Check sheet for the modelled part. Datum: model origin and axes. Units: mm. A direction names the side the tool comes from. Coordinates: 2 decimals unless noted, no trailing zeros. Loops run counter-clockwise (first coordinate to the right, second up) from the corner with the lowest first, then second, coordinate; pieces in that order, holes last. Notation, with made-up numbers: M 74,-19.75 L 89,-19.75 A17 ccw 89,-9.75 Z; hole C 41.25,51.25 d7. An arc over 180 degrees is marked long. Use CSV: the item, a comma, the result in double quotes. Start each with the question number.
(1) Go/stop test with flat-tipped pins: pin 1 Ø1.4 at (x, y) = (-67.5, -0.25) entering from -Z; pin 2 Ø1.5 at (x, z) = (-87.5, 3.5) entering from -Y; pin 3 Ø2.5 at (y, z) = (-21.5, 3) entering from -X; pin 4 Ø1.5 at (x, z) = (-59.5, 2.5) entering from -Y. Record where each tip stops, or that it passes through.
(2) Section check B-B on x = -64. Record the cut outline in (y, z), and give its area (3 significant figures).
(3) Set-up check for faces 1 (the flat face through (-34, -19.8, 2)), 2 (the flat face through (-1, 0, 5)), 3 (the flat face through (30, -22, 2)), 4 (the flat face through (-30.1, 22, 2)), 5 (the flat face through (82.45, -18, 2)): record each of +Z, -Z, +X, -X, +Y, -Y from which the full face is reachable in a straight line by a thin tool's end or side.
(4) Section check A-A on z = 2.4. Give the number of separate pieces and of enclosed holes in the cut face, and give its area (3 significant figures).
(5) Scan lines: line 1 (Y direction, x = 67.5, z = 3.9); line 2 (Y direction, x = -78, z = 0.7); line 3 (Y direction, x = -1.5, z = 1.85). Record each from-to range of solid material in increasing order.
Autodesk Inventor part; units mm, degrees
ref_plane "YZ Plane" through (0, 0, 0) normal (1, 0, 0) x (0, 1, 0)
ref_plane "XZ Plane" through (0, 0, 0) normal (0, 1, 0) x (-1, 0, 0)
ref_plane "XY Plane" through (0, 0, 0) normal (0, 0, 1) x (1, 0, 0)
sketch "Sketch1" plane through (0, 0, 0) normal (0, 0, 1) x (1, 0, 0)
  line L0 (-89.9, -25) -> (89.9, -25)
  line L1 (89.9, -25) -> (89.9, 25)
  line L2 (89.9, 25) -> (-89.9, 25)
  line L3 (-89.9, 25) -> (-89.9, -25)
  line L4 (-89.9, -25) -> (89.9, 25) construction
  line L5 (89.9, -25) -> (-89.9, 25) construction
  line L6 (46.5, 12.25) -> (67.5, 12.25) construction
  line L7 (67.5, 12.25) -> (67.5, -0.25) construction
  line L8 (67.5, -0.25) -> (46.5, -0.25) construction
  line L9 (46.5, -0.25) -> (46.5, 12.25) construction
  line L10 (46.5, 12.25) -> (67.5, -0.25) construction
  line L11 (67.5, 12.25) -> (46.5, -0.25) construction
  circle A0 centre (46.5, 12.25) radius 1.15
  circle A1 centre (67.5, 12.25) radius 1.15
  circle A2 centre (67.5, -0.25) radius 1.15
  circle A3 centre (46.5, -0.25) radius 1.15
  line L12 (-30.1, 25) -> (30.1, 25)
  line L13 (30.1, 25) -> (30.1, 20)
  line L14 (30.1, 20) -> (-30.1, 20)
  line L15 (-30.1, 20) -> (-30.1, 25)
  line L16 (-30.1, 25) -> (30.1, 20) construction
  line L17 (30.1, 25) -> (-30.1, 20) construction
  line L18 (-89.9, -19.8) -> (-30, -19.8)
  line L19 (-30, -19.8) -> (-30, -25)
  line L20 (-30, -25) -> (-89.9, -25)
  line L21 (-89.9, -25) -> (-89.9, -19.8)
  line L22 (-89.9, -19.8) -> (-30, -25) construction
  line L23 (-30, -19.8) -> (-89.9, -25) construction
  line L24 (19.7182, -25) -> (70.1, -25)
  line L25 (0, 0) -> (0, -25) construction
  line L26 (30, -25) -> (89.9, -25)
  line L27 (89.9, -25) -> (89.9, -19.8)
  line L28 (89.9, -19.8) -> (30, -19.8)
  line L29 (30, -19.8) -> (30, -25)
  line L30 (30, -25) -> (89.9, -19.8) construction
  line L31 (89.9, -25) -> (30, -19.8) construction
  line L32 (37.45, -16.8) -> (82.45, -16.8)
  line L33 (82.45, -16.8) -> (82.45, -19.8)
  line L34 (82.45, -19.8) -> (37.45, -19.8)
  line L35 (37.45, -19.8) -> (37.45, -16.8)
  line L36 (37.45, -16.8) -> (82.45, -19.8) construction
  line L37 (82.45, -16.8) -> (37.45, -19.8) construction
  point P0 (57, 6)
  point P1 (0, 22.5)
  point P2 (-59.95, -22.4)
  point P3 (30.1, 25)
  point P4 (-30.1, 25)
  point P5 (59.95, -22.4)
  point P6 (30, -25)
  point P7 (59.95, -18.3)
  point P8 (37.45, -19.8)
  dimension "d0" = 179.8
  dimension "d1" = 50
  dimension "d2" = 12.5
  dimension "d3" = 21
  dimension "d4" = 2.3
  dimension "d5" = 2.3
  dimension "d6" = 2.3
  dimension "d7" = 2.3
  dimension "d8" = 57
  dimension "d9" = 6
  dimension "d10" = 5
  dimension "d11" = 60.2
  dimension "d12" = 5.2
  dimension "d21" = 5.2
  dimension "d24" = 60
  dimension "d25" = 45
  dimension "d26" = 3
extrude "Extrusion1" add sketch "Sketch1" along normal blind 5 contours L19 L18 L3 L2 L15 L14 L13 L1 L28 L33 L32 L35 L29 L0 | L35 L32 L33 L28 | A0 | A1 | A2 | A3
extrude "Extrusion2" cut sketch "Sketch1" along normal through all contours L35 L32 L33 L28 | A0 | A1 | A2 | A3
mirror "Mirror1" about plane through (0, 0, 0) normal (1, 0, 0) of "Extrusion2"
equation "\"d5\" = d4"
equation "\"d6\" = d5"
equation "\"d7\" = d4"
properties part number "upper-front-plate-support" material "Glass"
Outcome:
1,pin 1,"passes through"
1,pin 2,"stops at y = -19.8"
1,pin 3,"stops at x = -30"
1,pin 4,"stops at y = -16.8"
2,outline,"M -16.8,0 L 25,0 L 25,5 L -16.8,5 Z"
2,area,"209 mm²"
3,face 1,"+Z, -Z, -X, -Y"
3,face 2,"+Z, +X, -X, +Y, -Y"
3,face 3,"+Z, -Z, +X, -Y"
3,face 4,"+Z, -Z, +Y"
3,face 5,"+Z, -Z, -Y"
4,separate pieces,"1"
4,enclosed holes,"8"
4,area,"7,760 mm²"
5,line 1,"y = -16.8 to -1.4, 0.9 to 11.1, 13.4 to 25"
5,line 2,"y = -16.8 to 25"
5,line 3,"y = -25 to 20"
